from build123d import *

# Parameters (mm, degrees)
F0_W        = 30
F0_H        = 30
F1_DEPTH    = 30
F2_R        = 5
F3_T1_DEPTH = 50
F3_T3_DEPTH = 55
F4_T1_DEPTH = 50
F4_T3_DEPTH = 55
F6_T1_DEPTH = 45


# Not quite as in the source:
# - a fillet or chamfer that OpenCascade refuses, or shapes differently, is made with other operations: its cross-section is extruded or revolved along the edge and cut away or added
# - a feature of the source that left no trace in its solid (it failed there, or was rolled back) is left out


with BuildPart() as f1:
    # F0 (on Right) → F1 (new body)
    with BuildSketch(Plane.YZ):
        with Locations((-5.478883007, 2.1195821464)):
            Rectangle(F0_W, F0_H)
    extrude(amount=F1_DEPTH)

    # F2
    f2_edges = [f1.edges().sort_by_distance(p)[0] for p in [
        (30, -5.478883, -12.880418),
        (30, 9.521117, 2.119582),
        (30, -5.478883, 17.119582),
        (30, -20.478883, 2.119582),
    ]]
    fillet(f2_edges, radius=F2_R)

    # F3: fillet of radius 5 on 4 edges, made by hand

    # F3_s2 → F3_t1 (cut)
    with BuildSketch(Plane.YZ.offset(-12.5)):
        with BuildLine():
            ThreePointArc((4.521116993, -12.8804178536), (8.0566508989, -11.4159517595), (9.521116993, -7.8804178536))
            Line((9.521116993, -7.8804178536), (9.521116993, -12.8804178536))
            Line((9.521116993, -12.8804178536), (4.521116993, -12.8804178536))
        make_face()
        with BuildLine():
            ThreePointArc((9.521116993, 12.1195821464), (8.0566508989, 15.6551160523), (4.521116993, 17.1195821464))
            Line((4.521116993, 17.1195821464), (9.521116993, 17.1195821464))
            Line((9.521116993, 17.1195821464), (9.521116993, 12.1195821464))
        make_face()
    extrude(amount=F3_T1_DEPTH, mode=Mode.SUBTRACT)

    # F3_s4 → F3_t3 (cut)
    with BuildSketch(Plane.XY.offset(-25.3804178536)):
        with BuildLine():
            ThreePointArc((0, 4.521116993), (1.4644660941, 8.0566508989), (5, 9.521116993))
            Line((5, 9.521116993), (0, 9.521116993))
            Line((0, 9.521116993), (0, 4.521116993))
        make_face()
    extrude(amount=F3_T3_DEPTH, mode=Mode.SUBTRACT)

    # F4: fillet of radius 5 on 4 edges, made by hand

    # F4_s2 → F4_t1 (cut)
    with BuildSketch(Plane.YZ.offset(-12.5)):
        with BuildLine():
            ThreePointArc((-20.478883007, 12.1195821464), (-19.0144169129, 15.6551160523), (-15.478883007, 17.1195821464))
            Line((-15.478883007, 17.1195821464), (-20.478883007, 17.1195821464))
            Line((-20.478883007, 17.1195821464), (-20.478883007, 12.1195821464))
        make_face()
        with BuildLine():
            ThreePointArc((-15.478883007, -12.8804178536), (-19.0144169129, -11.4159517595), (-20.478883007, -7.8804178536))
            Line((-20.478883007, -7.8804178536), (-20.478883007, -12.8804178536))
            Line((-20.478883007, -12.8804178536), (-15.478883007, -12.8804178536))
        make_face()
    extrude(amount=F4_T1_DEPTH, mode=Mode.SUBTRACT)

    # F4_s4 → F4_t3 (cut)
    with BuildSketch(Plane.XY.offset(-25.3804178536)):
        with BuildLine():
            ThreePointArc((5, -20.478883007), (1.4644660941, -19.0144169129), (0, -15.478883007))
            Line((0, -15.478883007), (0, -20.478883007))
            Line((0, -20.478883007), (5, -20.478883007))
        make_face()
    extrude(amount=F4_T3_DEPTH, mode=Mode.SUBTRACT)

    # F6: fillet of radius 5 on 4 edges, made by hand

    # F6_s2 → F6_t1 (cut)
    with BuildSketch(Plane.XZ.offset(-17.021116993)):
        with BuildLine():
            ThreePointArc((5, -12.8804178536), (1.4644660941, -11.4159517595), (0, -7.8804178536))
            Line((0, -7.8804178536), (0, -12.8804178536))
            Line((0, -12.8804178536), (5, -12.8804178536))
        make_face()
        with BuildLine():
            ThreePointArc((0, 12.1195821464), (1.4644660941, 15.6551160523), (5, 17.1195821464))
            Line((5, 17.1195821464), (0, 17.1195821464))
            Line((0, 17.1195821464), (0, 12.1195821464))
        make_face()
    extrude(amount=F6_T1_DEPTH, mode=Mode.SUBTRACT)


solid = f1.part
Can you work these out from the model? Positions are in its coordinate system, mm. Round coordinates to 2 decimals unless told otherwise and drop trailing zeros. Order: outer loops, then holes, each group sorted by start corner. A loop starts at its lowest first (then second) coordinate and runs counter-clockwise, first axis right, second up. Notation, with made-up numbers: (51.5, 26.25) -> (76.5, 26.25) arc R7 cw to (76.5, 30.25) -> close; hole circle Ø10 at (84, 52.25). An arc over 180 degrees is marked (long way). Write each question's results on one line, items separated by ' | '. Start each with the question number.
Item 1: If we section it at B-B, the plane z = 11: Write out the boundary of the cut face in (x, y), then the cut area to 3 significant figures.
Item 2: Please list where these lines run through material, in increasing order: L1, parallel to X at y = 7.5, z = 15; L2, parallel to X at y = 6, z = -1; L3, parallel to Z at x = 24, y = -17.5.
Item 3: Will this pin go through, and if not, where does the flat tip stop? pin 1 (1 mm diameter, centred on y = -5.5, z = 13, fed in from -X).
Item 4: Thinking about a two-plate mould opening in X: for faces 1 (the cylindrical face through (1.5, -5.29, -11.45)), 2 (the cylindrical face through (14.81, 8.02, -11.45)), 3 (the cylindrical face through (28.5, -5.29, 15.69)), which applies, +X half, -X half, draft (parallel to the pull), parting line (faces both ways), or undercut?
Item 5: If we section it at A-A, the plane x = 24: Write out the boundary of the cut face in (y, z).
Results:
1) outline: (0, -15.48) arc R5 ccw to (5, -20.48) -> (25, -20.48) arc R5 ccw to (30, -15.48) -> (30, 4.52) arc R5 ccw to (25, 9.52) -> (5, 9.52) arc R5 ccw to (0, 4.52) -> close | area: 879 mm2
2) L1: x = 0.98 to 29.02 | L2: x = 0.22 to 29.78 | L3: z = -12.45 to 16.69
3) pin 1: stops at x = 0.01
4) face 1: -X half | face 2: draft | face 3: +X half
5) outline: (-20.48, -7.88) arc R5 ccw to (-15.48, -12.88) -> (4.52, -12.88) arc R5 ccw to (9.52, -7.88) -> (9.52, 12.12) arc R5 ccw to (4.52, 17.12) -> (-15.48, 17.12) arc R5 ccw to (-20.48, 12.12) -> close
